Build history of the part. All positions in model axes, mm. A direction names the side the tool comes from. Round coordinates to 2 decimals unless told otherwise and drop trailing zeros. Loops run counter-clockwise (first coordinate to the right, second up) from the corner with the lowest first, then second, coordinate; pieces in that order, holes last. Notation, with made-up numbers: (74.25, 48.25) -> (102.25, 48.25) arc R19 ccw to (102.25, 53.25) -> close; hole circle Ø5 at (-36, 71). An arc over 180 degrees is marked (long way). Put each result on its own line as item: value. Start each with the question number.
```python
from build123d import *

# Parameters (mm, degrees)
ESBO_O1_W                = 107
ESBO_O1_H                = 25
ESBO_O1_R                = 3
RESSALTO_EXTRUS_O1_DEPTH = 3
ESBO_O1_11_W             = 12
ESBO_O1_11_H             = 2
ESBO_O1_11_W_2           = 10
ESBO_O1_11_W_3           = 25.5
ESBO_O1_11_W_4           = 2
ESBO_O1_11_H_2           = 6
ESBO_O1_11_H_3           = 9
RESSALTO_EXTRUS_O2_DEPTH = 20.5
ESBO_O1_12_W             = 12
ESBO_O1_12_H             = 2
ESBO_O1_12_W_2           = 2
ESBO_O1_12_H_2           = 6
RESSALTO_EXTRUS_O3_DEPTH = 23.5
ESBO_O1_13_R             = 3.5
RESSALTO_EXTRUS_O4_DEPTH = 5
ESBO_O1_14_R             = 1.5
CORTE_EXTRUS_O1_DEPTH    = 5
ESBO_O1_15_R             = 1.5
RESSALTO_EXTRUS_O5_DEPTH = 3


with BuildPart() as part:
    # Esboço1 → Ressalto-extrusão1 (new body)
    with BuildSketch(Plane.XY):
        with Locations((12.82231405, 20.771694215)):
            Rectangle(ESBO_O1_W, ESBO_O1_H)
        with BuildLine():
            Line((50.941584595, 12.8399279), (50.941584595, 26.5399279))
            ThreePointArc((50.941584595, 26.5399279), (58.441584595, 29.827875939), (65.941584595, 26.5399279))
            Line((65.941584595, 26.5399279), (65.941584595, 12.8399279))
            ThreePointArc((65.941584595, 12.8399279), (58.441584595, 9.518237762), (50.941584595, 12.8399279))
        make_face(mode=Mode.SUBTRACT)
        with Locations((-12.336122998, 19.452784517)):
            Circle(ESBO_O1_R, mode=Mode.SUBTRACT)
    extrude(amount=-RESSALTO_EXTRUS_O1_DEPTH)

    # Esboço1<11> → Ressalto-extrusão2 (add)
    with BuildSketch(Plane.XY):
        with Locations((50.32231405, 32.271694215)):
            Rectangle(ESBO_O1_11_W, ESBO_O1_11_H)
        with Locations((61.32231405, 32.271694215)):
            Rectangle(ESBO_O1_11_W_2, ESBO_O1_11_H)
        with Locations((31.57231405, 32.271694215)):
            Rectangle(ESBO_O1_11_W_3, ESBO_O1_11_H)
        with Locations((12.82231405, 32.271694215)):
            Rectangle(ESBO_O1_11_W, ESBO_O1_11_H)
        with Locations((-5.92768595, 32.271694215)):
            Rectangle(ESBO_O1_11_W_3, ESBO_O1_11_H)
        with Locations((-24.67768595, 32.271694215)):
            Rectangle(ESBO_O1_11_W, ESBO_O1_11_H)
        Polygon((-30.67768595, 33.271694215), (-40.67768595, 33.271694215), (-40.67768595, 31.271694215), (-38.67768595, 31.271694215), (-30.67768595, 31.271694215), align=None)
        with Locations((-39.67768595, 28.271694215)):
            Rectangle(ESBO_O1_11_W_4, ESBO_O1_11_H_2)
        with Locations((-39.67768595, 20.771694215)):
            Rectangle(ESBO_O1_11_W_4, ESBO_O1_11_H_3)
        with Locations((-39.67768595, 13.271694215)):
            Rectangle(ESBO_O1_11_W_4, ESBO_O1_11_H_2)
        with Locations((-39.67768595, 9.271694215)):
            Rectangle(ESBO_O1_11_W_4, ESBO_O1_11_H)
    extrude(amount=-RESSALTO_EXTRUS_O2_DEPTH)

    # Esboço1<12> → Ressalto-extrusão3 (add)
    with BuildSketch(Plane.XY):
        with Locations((50.32231405, 32.271694215)):
            Rectangle(ESBO_O1_12_W, ESBO_O1_12_H)
        with Locations((12.82231405, 32.271694215)):
            Rectangle(ESBO_O1_12_W, ESBO_O1_12_H)
        with Locations((-24.67768595, 32.271694215)):
            Rectangle(ESBO_O1_12_W, ESBO_O1_12_H)
        with Locations((-39.67768595, 28.271694215)):
            Rectangle(ESBO_O1_12_W_2, ESBO_O1_12_H_2)
        with Locations((-39.67768595, 13.271694215)):
            Rectangle(ESBO_O1_12_W_2, ESBO_O1_12_H_2)
    extrude(amount=-RESSALTO_EXTRUS_O3_DEPTH)

    # Esboço1<13> → Ressalto-extrusão4 (add)
    with BuildSketch(Plane.XY):
        with Locations((14.32231405, 15.171694215)):
            Circle(ESBO_O1_13_R)
        with Locations((31.82231405, 15.171694215)):
            Circle(ESBO_O1_13_R)
    extrude(amount=-RESSALTO_EXTRUS_O4_DEPTH)

    # Esboço1<14> → Corte-extrusão1 (cut)
    with BuildSketch(Plane.XY):
        with Locations((14.32231405, 15.171694215)):
            Circle(ESBO_O1_14_R)
        with Locations((31.82231405, 15.171694215)):
            Circle(ESBO_O1_14_R)
    extrude(amount=-CORTE_EXTRUS_O1_DEPTH, mode=Mode.SUBTRACT)

    # Esboço1<15> → Ressalto-extrusão5 (add)
    with BuildSketch(Plane.XY):
        with Locations((14.32231405, 15.171694215)):
            Circle(ESBO_O1_15_R)
        with Locations((31.82231405, 15.171694215)):
            Circle(ESBO_O1_15_R)
    extrude(amount=-RESSALTO_EXTRUS_O5_DEPTH)


solid = part.part
```
Item 1: Cut at A-A on x = 53.5. Write the cut outline in (y, z), then the cut area to 3 significant figures.
Item 2: Pull direction X, two halves, no side cores. Call faces 1 (the face through (12, 21, 0)), 2 (the face through (66.322, 24.4, -2.6)), 3 (the face through (50.942, 20, -1)): +X half, -X half, draft (parallel to the pull), parting line (faces both ways), or undercut.
Item 3: Drop flat-ended pins along their axis: pin 1 (1 mm diameter, centred on x = 61.5, y = 32.5, fed in from -Z); pin 2 (11.5 mm diameter, centred on x = 0, y = 14, fed in from -Z); pin 3 (3 mm diameter, centred on x = 51, z = -5, fed in from -Y). Give the stop position or say it passes through.
Item 4: Cut at B-B on z = -15.25. Write the cut outline in (x, y).
Item 5: Cut at C-C on x = -29.5. Write the cut outline in (y, z), then the cut area to 3 significant figures.
Item 6: 3-axis set-ups, long thin cutter, end or side, ignore diameter. For faces 4 (the face through (-40, 25.272, -22)), 5 (the face through (28.326, 15.326, -3.986)), 6 (the face through (16, 15, -5)), 7 (the face through (-36, 32, -20.5)): which of +Z, -Z, +X, -X, +Y, -Y reach the whole face in a straight line?
Item 7: Wall check: line 1 (Z direction, x = 0, y = 19.75); line 2 (X direction, y = 18, z = -19); line 3 (X direction, y = 17, z = -3.5). Give the ranges that are in metal, low to high. Write a range as from..to.
Ans:
1. outline: (8.27, -3) -> (10.81, -3) -> (10.81, 0) -> (8.27, 0) -> close; (28.55, -3) -> (31.27, -3) -> (31.27, -23.5) -> (33.27, -23.5) -> (33.27, 0) -> (28.55, 0) -> close
1. area: 62.8 mm2
2. face 1: draft
2. face 2: +X half
2. face 3: undercut
3. pin 1: stops at z = -20.5
3. pin 2: stops at z = -3
3. pin 3: stops at y = 31.27
4. outline: (-40.68, 8.27) -> (-38.68, 8.27) -> (-38.68, 31.27) -> (66.32, 31.27) -> (66.32, 33.27) -> (-40.68, 33.27) -> close
5. outline: (8.27, -3) -> (31.27, -3) -> (31.27, -23.5) -> (33.27, -23.5) -> (33.27, 0) -> (8.27, 0) -> close
5. area: 116 mm2
6. face 4: -Z, +X, -X
6. face 5: -Z
6. face 6: -Z, +X, -Y
6. face 7: -Z, -X, +Y
7. line 1: z = -3..0
7. line 2: x = -40.68..-38.68
7. line 3: x = -40.68..-38.68, 11.34..17.31, 28.84..34.81
